Model file for the job. Use its own axes, mm. Face numbers are marked on the shaded views. A direction names the side the tool comes from. Coordinates: 2 decimals unless noted, no trailing zeros. Loops run counter-clockwise (first coordinate to the right, second up) from the corner with the lowest first, then second, coordinate; pieces in that order, holes last.
from build123d import *

# Parameters (mm, degrees)
SKETCH1_W           = 19.1
SKETCH1_H           = 19.1
SKETCH1_W_2         = 14.1
SKETCH1_H_2         = 14.1
BOSS_EXTRUDE1_DEPTH = 4
SKETCH1_3_W         = 19.1
SKETCH1_3_H         = 19.1
SKETCH1_3_W_2       = 14.1
SKETCH1_3_H_2       = 14.1
BOSS_EXTRUDE2_DEPTH = 10
SKETCH2_R           = 2.625
BOSS_EXTRUDE3_DEPTH = 6
CHAMFER1_SIZE       = 0.1
FILLET1_R           = 0.5


with BuildPart() as part:
    # Sketch1 → Boss-Extrude1 (new body)
    # profile 1 of 2: a face of its own
    with BuildSketch(Plane(origin=(0, 0, 0), x_dir=(1, 0, 0), z_dir=(0, 1, 0))):
        with Locations((7.05, 7.05)):
            Rectangle(SKETCH1_W, SKETCH1_H)
        with Locations((7.05, 7.05)):
            Rectangle(SKETCH1_W_2, SKETCH1_H_2, mode=Mode.SUBTRACT)
    # profile 2 of 2: a face of its own
    with BuildSketch(Plane(origin=(0, 0, 0), x_dir=(1, 0, 0), z_dir=(0, 1, 0))):
        with Locations((7.05, 7.05)):
            Rectangle(SKETCH1_W_2, SKETCH1_H_2)
    extrude(amount=BOSS_EXTRUDE1_DEPTH)

    # Sketch1<3> → Boss-Extrude2 (add)
    with BuildSketch(Plane(origin=(0, 0, 0), x_dir=(1, 0, 0), z_dir=(0, 1, 0))):
        with Locations((7.05, 7.05)):
            Rectangle(SKETCH1_3_W, SKETCH1_3_H)
        with Locations((7.05, 7.05)):
            Rectangle(SKETCH1_3_W_2, SKETCH1_3_H_2, mode=Mode.SUBTRACT)
    extrude(amount=BOSS_EXTRUDE2_DEPTH)

    # Sketch2 → Boss-Extrude3 (add)
    with BuildSketch(Plane(origin=(0, 4, 0), x_dir=(1, 0, 0), z_dir=(0, 1, 0))):
        with Locations(Location((7.05, 7.05, 0), (0, 0, 90))):
            Circle(SKETCH2_R)
        with BuildLine():
            Line((6.15, 6.45), (4.975, 6.45))
            Line((4.975, 6.45), (4.975, 7.65))
            Line((4.975, 7.65), (6.15, 7.65))
            ThreePointArc((6.15, 7.65), (6.362132034, 7.737867966), (6.45, 7.95))
            Line((6.45, 7.95), (6.45, 9.125))
            Line((6.45, 9.125), (7.65, 9.125))
            Line((7.65, 9.125), (7.65, 7.95))
            ThreePointArc((7.65, 7.95), (7.737867966, 7.737867966), (7.95, 7.65))
            Line((7.95, 7.65), (9.125, 7.65))
            Line((9.125, 7.65), (9.125, 6.45))
            Line((9.125, 6.45), (7.95, 6.45))
            ThreePointArc((7.95, 6.45), (7.737867966, 6.362132034), (7.65, 6.15))
            Line((7.65, 6.15), (7.65, 4.975))
            Line((7.65, 4.975), (6.45, 4.975))
            Line((6.45, 4.975), (6.45, 6.15))
            ThreePointArc((6.45, 6.15), (6.362132034, 6.362132034), (6.15, 6.45))
        make_face(mode=Mode.SUBTRACT)
    extrude(amount=BOSS_EXTRUDE3_DEPTH)

    # Chamfer1
    chamfer1_edges = [part.edges().sort_by_distance(p)[0] for p in [
        (5.5625, 10, -6.45),
        (7.05, 10, -9.125),
        (7.65, 10, -8.5375),
        (9.125, 10, -7.05),
        (8.5375, 10, -6.45),
        (7.65, 10, -5.5625),
        (7.05, 10, -4.975),
        (6.45, 10, -5.5625),
        (6.362132034, 10, -6.362132034),
        (4.975, 10, -7.05),
        (5.5625, 10, -7.65),
        (6.362132034, 10, -7.737867966),
        (6.45, 10, -8.5375),
        (7.737867966, 10, -7.737867966),
        (8.5375, 10, -7.65),
        (7.737867966, 10, -6.362132034),
    ]]
    chamfer(chamfer1_edges, length=CHAMFER1_SIZE)

    # Fillet1
    fillet1_edges = [part.edges().sort_by_distance(p)[0] for p in [
        (-2.5, 5, -16.6),
        (16.6, 5, -16.6),
        (16.6, 5, 2.5),
        (-2.5, 5, 2.5),
    ]]
    fillet(fillet1_edges, radius=FILLET1_R)


solid = part.part
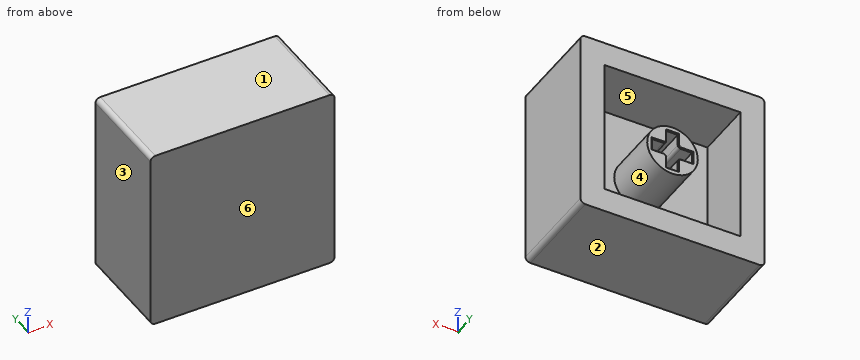
Q1. Which spindle directions (+Z, -Z, +X, -X, +Y, -Y) get a long thin tool onto all of the face, cutting with end or side? Do the marked faces 5 and 6. Say none if no direction does.
Answers:
face 5: +Y
face 6: +Z, -Z, +X, -X, -Y
Q2. Slice it at C-C (z = -0.5). List the corners of the cut face in (x, y).
Answers:
outline: (-2.5, 0) - (16.6, 0) - (16.6, 10) - (14.1, 10) - (14.1, 4) - (0, 4) - (0, 10) - (-2.5, 10) - close
Q3. Slice it at D-D (z = -7.05). List the corners of the cut face in (x, y) (3 decimals).
Answers:
outline: (-2.5, 0) - (16.6, 0) - (16.6, 10) - (14.1, 10) - (14.1, 4) - (9.675, 4) - (9.675, 10) - (9.225, 10) - (9.125, 9.9) - (9.125, 4) - (4.975, 4) - (4.975, 9.9) - (4.875, 10) - (4.425, 10) - (4.425, 4) - (0, 4) - (0, 10) - (-2.5, 10) - close
Q4. Slice it at B-B (x = 0.75). List the corners of the cut face in (y, z), and give its area (3 significant figures).
Answers:
outline: (0, -16.6) - (10, -16.6) - (10, -14.1) - (4, -14.1) - (4, 0) - (10, 0) - (10, 2.5) - (0, 2.5) - close
area: 106 mm2
Q5. Drill centre lines: line 1 (Z direction, x = 8.5, y = 4.25); line 2 (Z direction, x = 13, y = 9); line 3 (X direction, y = 7.75, z = -5.75). Where is each one in solid material? Low to high.
Answers:
line 1: z = -16.6 to -14.1, -9.24 to -7.65, -6.45 to -4.86, 0 to 2.5
line 2: z = -16.6 to -14.1, 0 to 2.5
line 3: x = -2.5 to 0, 4.77 to 6.45, 7.65 to 9.33, 14.1 to 16.6
Q6. Slice it at A-A (y = 7). Count the separate pieces of the cut face and the enclosed holes in it, and give its area (3 significant figures).
Answers:
separate pieces: 2
enclosed holes: 2
area: 179 mm2
Q7. Mould opens along Z. For the marked faces 1, 2, 3 and 4 say: +Z half, -Z half, draft (parallel to the pull), parting line (faces both ways), or undercut.
Answers:
face 1: +Z half
face 2: -Z half
face 3: draft
face 4: undercut
